from build123d import *

# Parameters (mm, degrees)
EXTRUDE_1_DEPTH = 4
SKETCH_2_R      = 3
EXTRUDE_2_DEPTH = 10
CHAMFER_1_SIZE  = 1


with BuildPart() as part:
    # Эскиз1 → Вытянуть1 (new body)
    with BuildSketch(Plane.XY):
        Polygon((0, 5.773502692), (-5, 2.886751346), (-5, -2.886751346), (0, -5.773502692), (5, -2.886751346), (5, 2.886751346), align=None)
    extrude(amount=EXTRUDE_1_DEPTH)

    # Эскиз2 → Вытянуть2 (add)
    with BuildSketch(Plane(origin=(0, 0, 0), x_dir=(-1, 0, 0), z_dir=(0, 0, -1))):
        with Locations(Location((0, 0, 0), (0, 0, 180))):
            Circle(SKETCH_2_R)
    extrude(amount=EXTRUDE_2_DEPTH)

    # Эскиз15 → Вырез-Повернуть1 (revolve, cut)
    with BuildSketch(Plane(origin=(0, 0, 0), x_dir=(0, 0, -1), z_dir=(1, 0, 0)), mode=Mode.PRIVATE) as cut_revolve_1_sk:
        Polygon((-4, 5.773502692), (-4, 4.973502692), (-3.2, 5.773502692), align=None)
    revolve(cut_revolve_1_sk.sketch.rotate(Axis((0, 0, 2.465296569), (0, 0, -1)), 300.000000095), axis=Axis((0, 0, 2.465296569), (0, 0, -1)), mode=Mode.SUBTRACT)

    # Фаска1
    chamfer_1_edges = [part.edges().sort_by_distance(p)[0] for p in [
        (-3, 0, -10),
    ]]
    chamfer(chamfer_1_edges, length=CHAMFER_1_SIZE)


solid = part.part
Part model, mm, in its own coordinate system. A direction names the side the tool comes from. Give positions to 0.01 mm unless a question says otherwise; leave off trailing zeros. Order: outer loops, then holes, each group sorted by start corner. A loop starts at its lowest first (then second) coordinate and runs counter-clockwise, first axis right, second up. Notation, with made-up numbers: (46, 42) - (54, 42) arc R12 cw to (54, 60) - close; hole circle Ø10 at (-29, 81.25). An arc over 180 degrees is marked (long way). One line per question, with ' | ' between items.
1. Which spindle directions (+Z, -Z, +X, -X, +Y, -Y) get a long thin tool onto all of the face, cutting with end or side? Do faces 1 (the face through (2.2, -2.5, 0)), 2 (the face through (5, 0, 2)). Say none if no direction does.
Filled in:
face 1: -Z | face 2: +Z, -Z, +X, +Y, -Y
2. Drop flat-ended pins along their axis: P1, Ø2, axis at x = -2, z = -3, coming from the -Y side; P2, Ø1, axis at x = -1, y = -3, coming from the -Z side. Give the stop position or say it passes through.
Filled in:
P1: y = -2.83 | P2: z = -9.34
3. Band-saw the part on B-B on z = 1. List the corners of the cut face in (x, y), then the cut area to 3 significant figures.
Filled in:
outline: (-5, -2.89) - (0, -5.77) - (5, -2.89) - (5, 2.89) - (0, 5.77) - (-5, 2.89) - close | area: 86.6 mm²
4. Drill centre lines: probe 1 along Z at (x, y) = (-2.75, -3); probe 2 along X at (y, z) = (-1.25, -7.5); probe 3 along Y at (x, z) = (3.75, 0.75). Where is each one in solid material? Low to high.
Filled in:
probe 1: 0 to 4 | probe 2: -2.73 to 2.73 | probe 3: -3.61 to 3.61
5. Band-saw the part on C-C on z = -3. List the corners of the cut face in (x, y), then the cut area to 3 significant figures.
Filled in:
outline: circle Ø6 at (0, 0) | area: 28.3 mm²
